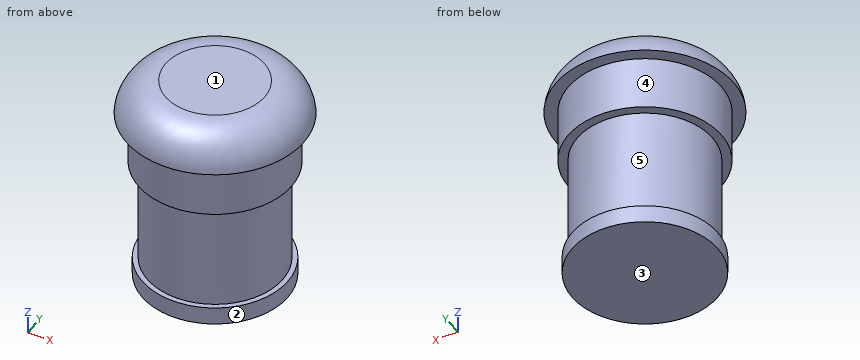
Autodesk Inventor part; units mm, degrees
ref_plane "YZ Plane" through (0, 0, 0) normal (1, 0, 0) x (0, 1, 0)
ref_plane "XZ Plane" through (0, 0, 0) normal (0, 1, 0) x (-1, 0, 0)
ref_plane "XY Plane" through (0, 0, 0) normal (0, 0, 1) x (1, 0, 0)
sketch "Sketch1" plane through (0, 0, 0) normal (0, 0, 1) x (1, 0, 0)
  circle A0 centre (0, 0) radius 20.32
  dimension "d0" = 40.64
extrude "Extrusion1" add sketch "Sketch1" along normal blind 5
sketch "Sketch2" plane through (0, 0, 5) normal (0, 0, 1) x (1, 0, 0)
  circle A0 centre (0, 0) radius 18.8864
extrude "Extrusion4" add sketch "Sketch2" along normal blind 30
sketch "Sketch3" plane through (0, 0, 35) normal (0, 0, 1) x (1, 0, 0)
  circle A0 centre (0, 0) radius 21.3705
extrude "Extrusion5" add sketch "Sketch3" along normal blind 15
sketch "Sketch4" plane through (0, 0, 50) normal (0, 0, 1) x (1, 0, 0)
  circle A0 centre (0, 0) radius 24.7853
extrude "Extrusion6" add sketch "Sketch4" along normal blind 10
fillet "Fillet1" radius 11 1 edges at (-24.7853, 0, 60)
equation "\"BendRadius\" = Thickness"
equation "\"BendReliefWidth\" = Thickness"
equation "\"BendReliefDepth\" = 0.5 * Thickness"
equation "\"CornerReliefSize\" = 4 * Thickness"
equation "\"MinimumRemnant\" = 2 * Thickness"
equation "\"TransitionRadius\" = BendRadius"
equation "\"JacobiRadiusSize\" = BendRadius"
equation "\"GapSize\" = Thickness"
properties part number "hitan_stop"
Read the model definition and answer for the solid it produces. Units are mm, in the model's axes. Face numbers are marked on the shaded views. A direction names the side the tool comes from. Coordinates: 2 decimals unless noted, no trailing zeros. Write each loop counter-clockwise with the first axis right and the second up, starting at its lowest first coordinate (ties: lowest second). Pieces come first, ordered by that corner, then holes. Notation, with made-up numbers: (87.25, -38) -> (140.25, -38) arc R29 ccw to (140.25, -17) -> close; hole circle Ø7 at (-13, 75). An arc over 180 degrees is marked (long way). Return JSON: item names as keys, results as strings.
(1) The part is cut by section D-D on z = 51.5. Give the vertices of the cut face in (x, y).
Answers below:
{"outline": "circle Ø49.09 at (0, 0)"}
(2) The part is cut by section C-C on z = 25.5. Give the vertices of the cut face in (x, y), then the cut area to 3 significant figures.
Answers below:
{"outline": "circle Ø37.77 at (0, 0)", "area": "1,120 mm^2"}
(3) Which of the six approach directions +Z, -Z, +X, -X, +Y, -Y give full straight-line access (tool end or side, diameter ignored) to the marked faces 1 and 2?
Answers below:
{"face 1": "+Z, +X, -X, +Y, -Y", "face 2": "-Z"}
(4) Consider line 1 along Z through (x, y) = (4, -18.5); line 2 along Y through (x, z) = (-3, 47); line 3 along X through (y, z) = (6, 41). Determine where each line is inside the solid, lowest interval first. Write a range as from..to.
Answers below:
{"line 1": "0..5, 35..58.75", "line 2": "-21.16..21.16", "line 3": "-20.51..20.51"}
(5) Each of these flat-tipped pins is pushed along its axis until it touches: P1, Ø1.5, axis at y = -7, z = 51, coming from the +X side; P2, Ø2, axis at x = -7, y = 17, coming from the +Z side; P3, Ø12, axis at x = 15.5, z = 10.5, coming from the +Y side. Where does it stop, or does it pass through?
Answers below:
{"P1": "x = 23.88", "P2": "z = 59.41", "P3": "y = 16.32"}
(6) The part is cut by section A-A on x = 0. Give the vertices of the cut face in (y, z).
Answers below:
{"outline": "(-24.79, 50) -> (-21.37, 50) -> (-21.37, 35) -> (-18.89, 35) -> (-18.89, 5) -> (-20.32, 5) -> (-20.32, 0) -> (20.32, 0) -> (20.32, 5) -> (18.89, 5) -> (18.89, 35) -> (21.37, 35) -> (21.37, 50) -> (24.79, 50) arc R11 ccw to (13.83, 60) -> (-13.83, 60) arc R11 ccw to start"}
(7) For a pull along Z with two mould halves and no side action, classify the marked faces 3, 4 and 5 as pulls with the +Z half, pulls with the -Z half, needs draft (parallel to the pull), parting line crosses it, or undercut.
Answers below:
{"face 3": "pulls with the -Z half", "face 4": "needs draft", "face 5": "undercut"}
